from build123d import *

# Parameters (mm, degrees)
F0_W     = 130.64453
F0_H     = 211.371556
F1_DEPTH = 374.337018
F2_T     = -2.54


with BuildPart() as f1:
    # F0 (on Front) → F1 (new body)
    with BuildSketch(Plane.XZ):
        with Locations((65.322265, 105.685778)):
            Rectangle(F0_W, F0_H)
    extrude(amount=F1_DEPTH)

    # F2
    f2_openings = [f1.faces().sort_by_distance(p)[0] for p in [
        (65.322265, -374.337018, 105.685778),
        (65.322265, -187.168509, 211.371556),
    ]]
    offset(amount=F2_T, openings=f2_openings)


solid = f1.part
Design review of the part built by this model. Coordinates are the model's own, in mm. A direction names the side the tool comes from. Give positions to 0.01 mm unless a question says otherwise; leave off trailing zeros. Loops run counter-clockwise (first coordinate to the right, second up) from the corner with the lowest first, then second, coordinate; pieces in that order, holes last. Notation, with made-up numbers: (40, 44) -> (59, 44) arc R18 cw to (59, 60) -> close; hole circle Ø6 at (87.5, -35.75). An arc over 180 degrees is marked (long way). One line per question, with ' | ' between items. Start each with the question number.
(1) For line 1 (X direction, y = -212, z = 115); line 2 (Z direction, x = 103.5, y = -269.5); line 3 (Y direction, x = 20.5, z = 30.5), list the stretches that pass through material, from the lowest coordinate up.
(2) We need section B-B (z = 134). State the section outline as (x, y) points.
(3) Insertion check: P1, Ø5, axis at x = 106, z = 167, coming from the +Y side; P2, Ø1.5, axis at x = 57.5, y = -231, coming from the +Z side; P3, Ø8, axis at x = 73, z = 135.5, coming from the -Y side. Each pin has a flat end and moves straight along its axis. Give the tip position at first contact, or say it passes through.
(4) We need section C-C (x = 85). State the section outline as (y, z) points, and give its area (3 significant figures).
(5) We need section A-A (y = -282). State the section outline as (x, z) points.
(6) For faces 1 (the face through (130.645, -185, 104)), 2 (the face through (64, -2.54, 108)), list the 3-axis set-ups (+Z, -Z, +X, -X, +Y, -Y) from which the entire face can be reached by the end or side of a thin tool; tool diameter is ignored.
The answers:
1) line 1: x = 0 to 2.54, 128.1 to 130.64 | line 2: z = 0 to 2.54 | line 3: y = -2.54 to 0
2) outline: (0, -374.34) -> (2.54, -374.34) -> (2.54, -2.54) -> (128.1, -2.54) -> (128.1, -374.34) -> (130.64, -374.34) -> (130.64, 0) -> (0, 0) -> close
3) P1: stops at y = 0 | P2: stops at z = 2.54 | P3: stops at y = -2.54
4) outline: (-374.34, 0) -> (0, 0) -> (0, 211.37) -> (-2.54, 211.37) -> (-2.54, 2.54) -> (-374.34, 2.54) -> close | area: 1,480 mm^2
5) outline: (0, 0) -> (130.64, 0) -> (130.64, 211.37) -> (128.1, 211.37) -> (128.1, 2.54) -> (2.54, 2.54) -> (2.54, 211.37) -> (0, 211.37) -> close
6) face 1: +Z, -Z, +X, +Y, -Y | face 2: +Z, -Y
